For this review, use the dimensioned drawing (mm, ordinates from the lowest corner) and the shaded views. Give positions to 0.01 mm unless a question says otherwise; leave off trailing zeros. Loops run counter-clockwise (first coordinate to the right, second up) from the corner with the lowest first, then second, coordinate; pieces in that order, holes last. Notation, with made-up numbers: M -9,-6 L 44,-6 A18 ccw 44,18 Z; hole C -11.5,29 d9. An arc over 180 degrees is marked long. Use one line per item in the form item = value. Start each with the question number.
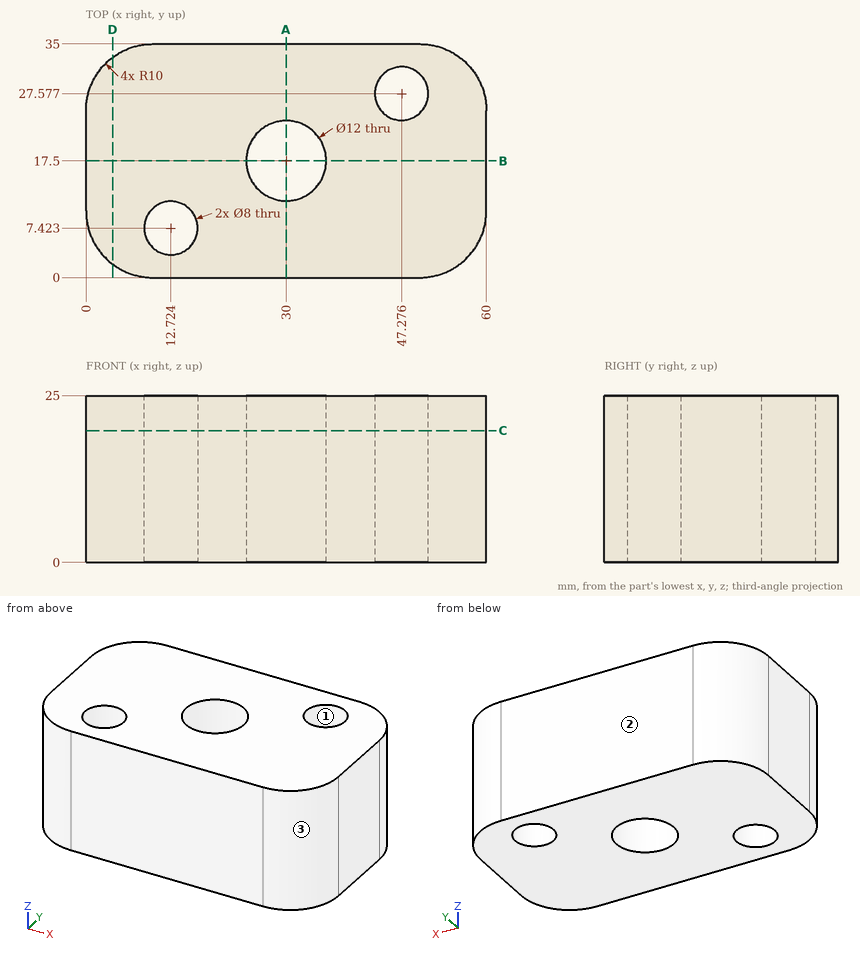
Q1. Wall thickness on probe 1 along Y at (x, z) = (13, 21.75); probe 2 along Y at (x, z) = (49, 14.25) (1 decimal); probe 3 along X at (y, z) = (13, 12.25): over which ranges is each line inside the solid? List them lowest first.
Q2. Take a section at C-C on z = 19.75. Give the boundary of the cut face in (x, y) (1 decimal), plus the area to 3 significant figures.
Q3. The part is to be moulded in two halves that separate along X. For the marked faces 1, 2 and 3, say which applies: pulls with the +X half, pulls with the -X half, needs draft (parallel to the pull), parting line crosses it, or undercut.
Q4. Take a section at A-A on x = 30. Give the boundary of the cut face in (y, z), plus the area to 3 significant figures.
Q5. Take a section at B-B on y = 17.5. Give the boundary of the cut face in (x, z).
Q6. Clearance check with flat-ended pins moving along their axes: pin 1 Ø15.5 at (x, y) = (30, 17.5) entering from -Z; pin 2 Ø1 at (x, y) = (30.5, 21.5) entering from -Z; pin 3 Ø3 at (y, z) = (4, 22.5) entering from -X. State where each tip first meets the part, or that it passes through.
Q7. Take a section at D-D on x = 4. Give the boundary of the cut face in (y, z).
Response values:
q1.probe_1 = 0 to 3.43, 11.41 to 35
q1.probe_2 = 0 to 24, 31.2 to 35
q1.probe_3 = 0 to 26.03, 33.97 to 60
q2.outline = M 0,10 A10 ccw 10,0 L 50,0 A10 ccw 60,10 L 60,25 A10 ccw 50,35 L 10,35 A10 ccw 0,25 Z; hole C 12.7,7.4 d8; hole C 30,17.5 d12; hole C 47.3,27.6 d8
q2.area = 1,800 mm^2
q3.face_1 = undercut
q3.face_2 = needs draft
q3.face_3 = pulls with the +X half
q4.outline = M 0,0 L 11.5,0 L 11.5,25 L 0,25 Z; M 23.5,0 L 35,0 L 35,25 L 23.5,25 Z
q4.area = 575 mm^2
q5.outline = M 0,0 L 24,0 L 24,25 L 0,25 Z; M 36,0 L 60,0 L 60,25 L 36,25 Z
q6.pin_1 = 0
q6.pin_2 = through
q6.pin_3 = 1.07
q7.outline = M 2,0 L 33,0 L 33,25 L 2,25 Z
